Answer from the drawing. Dimensions are ordinates in mm from the lowest x, y and z of the part. A direction names the side the tool comes from. Round coordinates to 2 decimals unless told otherwise and drop trailing zeros. Write each loop counter-clockwise with the first axis right and the second up, starting at its lowest first coordinate (ties: lowest second). Pieces come first, ordered by that corner, then holes. Notation, with made-up numbers: (73, 82.25) -> (122, 82.25) arc R29 ccw to (122, 120.25) -> close; hole circle Ø4 at (-21, 33). An arc over 180 degrees is marked (long way). Return JSON: item names as keys, results as strings. Group by question number.
(1) The mould has two halves that part along X. Classify the marked faces 1, 2, 3 and 4: released by +X, released by -X, zero draft, split by the parting line, or undercut.
(2) A cutting plane is placed at C-C on y = 3.5. Give the vertices of the cut face in (x, z).
(3) For the marked faces 5, 6 and 7, determine the directions among +Z, -Z, +X, -X, +Y, -Y from which every point of the face is accessible in a straight line to the end or side of a thin tool.
(4) Straight lines are drawn through the part: line 1 (Z direction, x = 12.35, y = 3.5); line 2 (Z direction, x = 12.35, y = 6.75); line 3 (X direction, y = 5.25, z = 12) (1 decimal). For each, find the intervals that lie inside material, in ascending order.
(5) A cutting plane is placed at A-A on z = 4. Give the vertices of the cut face in (x, y).
(6) Given pin 1 (2 mm diameter, centred on x = 15.5, y = 7, fed in from +Z); pin 2 (4 mm diameter, centred on y = 7, z = 10.5, fed in from +X) (1 decimal); pin 3 (1.1 mm diameter, centred on y = 6, z = 13.5, fed in from -X) (1 decimal), each flat-ended and moving along its own axis, determine where each tip first touches the part or whether it passes through.
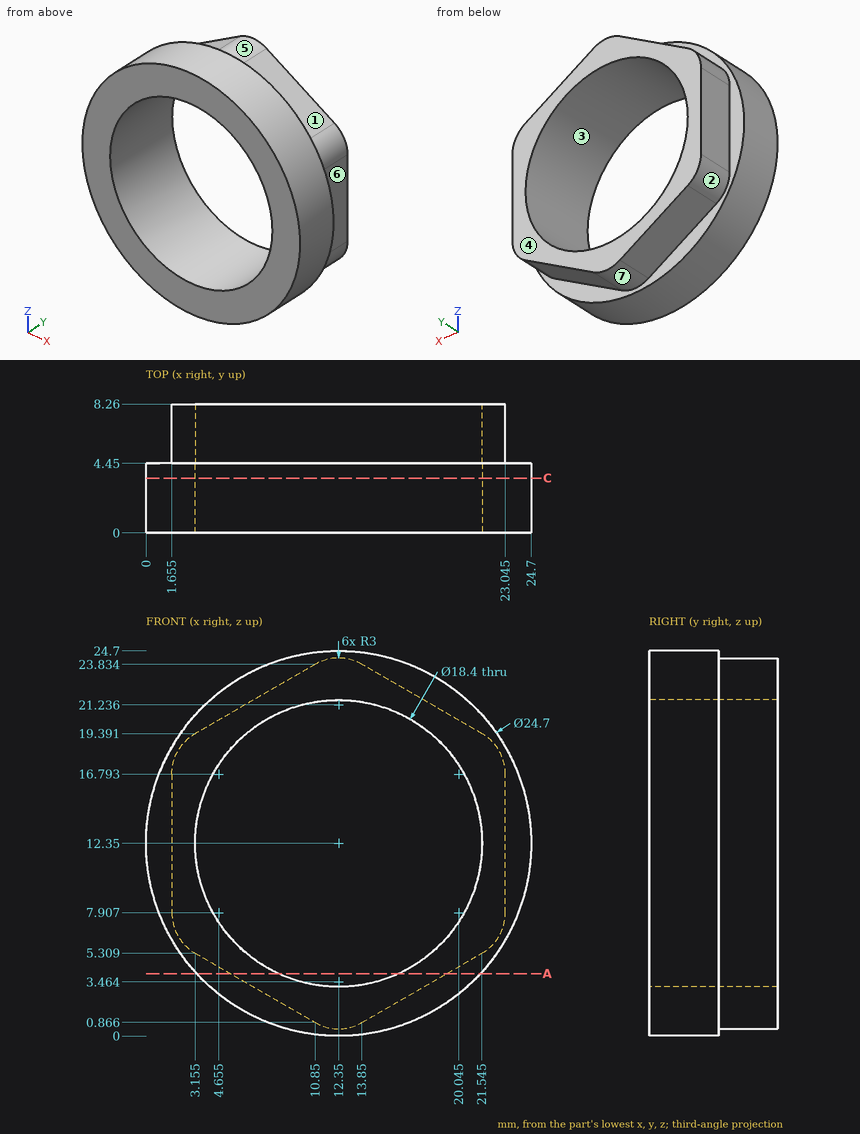
Checks:
{
 "1": {"face 1": "released by +X", "face 2": "released by -X", "face 3": "undercut", "face 4": "zero draft"},
 "2": {"outline": "circle Ø24.7 at (12.35, 12.35); hole circle Ø18.4 at (12.35, 12.35)"},
 "3": {"face 5": "+Z, +Y", "face 6": "+Z, -Z, +X, +Y", "face 7": "-Z, +Y"},
 "4": {"line 1": "z = 0 to 3.15, 21.55 to 24.7", "line 2": "z = 0.46 to 3.15, 21.55 to 24.24", "line 3": "x = 1.7 to 3.2, 21.5 to 23"},
 "5": {"outline": "(3.25, 0) -> (8.49, 0) -> (8.49, 8.26) -> (5.42, 8.26) -> (5.42, 4.45) -> (3.25, 4.45) -> close; (16.21, 0) -> (21.45, 0) -> (21.45, 4.45) -> (19.28, 4.45) -> (19.28, 8.26) -> (16.21, 8.26) -> close"},
 "6": {"pin 1": "stops at z = 23.46", "pin 2": "stops at x = 23", "pin 3": "stops at x = 1.7"}
}
